```python
from build123d import *

# Parameters (mm, degrees)
BOSS_EXTRUDE1_DEPTH = 12
BOSS_EXTRUDE2_DEPTH = 13
SKETCH3_W           = 9
SKETCH3_H           = 12
BOSS_EXTRUDE3_DEPTH = 3.3
CUT_EXTRUDE1_DEPTH  = 34.256578297
CUT_EXTRUDE2_DEPTH  = 25.143114961
CUT_EXTRUDE3_DEPTH  = 25.143114961
CUT_EXTRUDE4_DEPTH  = 28.6007146
CUT_EXTRUDE5_DEPTH  = 28.748873851
CHAMFER1_SIZE       = 2.129646437


with BuildPart() as part:
    # Sketch1 → Boss-Extrude1 (new body)
    with BuildSketch(Plane.XZ.offset(17)):
        Polygon((16, 15), (3.3, 15), (3.3, 6), (11.968992121, -12.590713597), (16, -12.590713597), align=None)
    extrude(amount=-BOSS_EXTRUDE1_DEPTH)

    # Sketch2 → Boss-Extrude2 (add)
    with BuildSketch(Plane(origin=(0, -5, 0), x_dir=(-1, 0, 0), z_dir=(0, 1, 0))):
        Polygon((-16, 15), (-3.3, 15), (-3.3, 6), (-6.717465771, -1.328778996), (-13.611865759, -7.113867483), (-16, -4.267799921), align=None)
    extrude(amount=BOSS_EXTRUDE2_DEPTH)

    # Sketch3 → Boss-Extrude3 (add)
    with BuildSketch(Plane.ZY.offset(-3.3)):
        with Locations((10.5, -11)):
            Rectangle(SKETCH3_W, SKETCH3_H)
    extrude(amount=BOSS_EXTRUDE3_DEPTH)

    # Sketch4 → Cut-Extrude1 (cut, through all)
    with BuildSketch(Plane.XZ.offset(17)):
        Polygon((16, 15), (8.3, 15), (8.3, 3.870353563), (16, -2.590713597), align=None)
    extrude(amount=-CUT_EXTRUDE1_DEPTH, mode=Mode.SUBTRACT)

    # Sketch5 → Cut-Extrude2 (cut, through all)
    with BuildSketch(Plane(origin=(8.3, 0, 0), x_dir=(0, 0, -1), z_dir=(1, 0, 0))):
        with BuildLine():
            Line((-8.917452439, -10.971751585), (-10.5, -9.332975613))
            Line((-10.5, -9.332975613), (-12.082547561, -10.971751585))
            ThreePointArc((-12.082547561, -10.971751585), (-10.5, -14.7), (-8.917452439, -10.971751585))
        make_face()
    extrude(amount=-CUT_EXTRUDE2_DEPTH, mode=Mode.SUBTRACT)

    # Sketch6 → Cut-Extrude3 (cut, through all)
    with BuildSketch(Plane(origin=(8.3, 0, 0), x_dir=(0, 0, -1), z_dir=(1, 0, 0))):
        with BuildLine():
            Line((-8.917452439, 4.028248415), (-10.5, 5.667024387))
            Line((-10.5, 5.667024387), (-12.082547561, 4.028248415))
            ThreePointArc((-12.082547561, 4.028248415), (-10.5, 0.3), (-8.917452439, 4.028248415))
        make_face()
    extrude(amount=-CUT_EXTRUDE3_DEPTH, mode=Mode.SUBTRACT)

    # Sketch7 → Cut-Extrude4 (cut, through all)
    with BuildSketch(Plane(origin=(5.33513716, 0, 6.358168878), x_dir=(0.766044443118978, 0, -0.6427876096865394), z_dir=(0.6427876096865394, 0, 0.766044443118978))):
        with BuildLine():
            Line((12.082582782, 4.028248415), (10.500035221, 5.667024387))
            Line((10.500035221, 5.667024387), (8.91748766, 4.028248415))
            ThreePointArc((8.91748766, 4.028248415), (10.500035221, 0.3), (12.082582782, 4.028248415))
        make_face()
    extrude(amount=-CUT_EXTRUDE4_DEPTH, mode=Mode.SUBTRACT)

    # Sketch8 → Cut-Extrude5 (cut, through all)
    with BuildSketch(Plane(origin=(16, 0, 0), x_dir=(0, 0, -1), z_dir=(1, 0, 0))):
        with BuildLine():
            Line((9.852318341, -8.471751585), (8.26977078, -6.832975613))
            Line((8.26977078, -6.832975613), (6.68722322, -8.471751585))
            ThreePointArc((6.68722322, -8.471751585), (8.26977078, -12.2), (9.852318341, -8.471751585))
        make_face()
    extrude(amount=-CUT_EXTRUDE5_DEPTH, mode=Mode.SUBTRACT)

    # Chamfer1
    chamfer1_edges = [part.edges().sort_by_distance(p)[0] for p in [
        (8.3, -4.5, 3.870353563),
    ]]
    chamfer(chamfer1_edges, length=CHAMFER1_SIZE)


solid = part.part
```
Geometry check sheet. Reference: the model listing, model coordinates, mm. A direction names the side the tool comes from. Coordinates: 2 decimals unless noted, no trailing zeros. Write each loop counter-clockwise with the first axis right and the second up, starting at its lowest first coordinate (ties: lowest second). Pieces come first, ordered by that corner, then holes. Notation, with made-up numbers: M -26.5,37 L 4.5,37 A34 ccw 4.5,68 Z; hole C 84.5,15 d6. An arc over 180 degrees is marked long. Use one line per item in the form item = value. Start each with the question number.
1) Section check B-B on y = -3.75. Enter the section's corners in (x, z), and give its area (3 significant figures).
2) Thickness scan on probe 1 along Z at (x, y) = (12, -10); probe 2 along X at (y, z) = (-13.5, 8); probe 3 along Z at (x, y) = (11.5, -8.5). Record the ranges inside material, lowest first. Write a range as from..to.
3) Section check D-D on y = -13.75. Enter the section's corners in (x, z).
4) Go/stop test with flat-tipped pins: pin 1 Ø4.5 at (y, z) = (3.5, 9) entering from -X; pin 2 Ø1 at (x, y) = (5, 4.5) entering from -Z; pin 3 Ø3 at (x, z) = (12, -10) entering from +Y; pin 4 Ø3.5 at (y, z) = (-10, -8.27) entering from -X. Record where each tip stops, or that it passes through.
5) Release check for a two-part mould opening along Y. For faces 1 (the flat face through (4.21, -10.14, 11.28)), 2 (the flat face through (8, 8, 4)), 3 (the flat face through (0, -9.6, 11.4)) record: pulls with the +Y half, pulls with the -Y half, needs draft (parallel to the pull), parting line crosses it, or undercut.
6) Section check A-A on x = 3.75. Enter the section's corners in (y, z).
7) Section check C-C on y = 1. Enter the section's corners in (x, z).
8) Set-up check for faces 4 (the flat face through (14.8, 1.4, -5.7)), 5 (the flat face through (5.84, 4.84, 9.7)), 6 (the flat face through (2, -11, 6)): record each of +Z, -Z, +X, -X, +Y, -Y from which the full face is reachable in a straight line by a thin tool's end or side.
Responses:
q1.outline = M 3.3,6 L 6.72,-1.33 L 13.61,-7.11 L 16,-4.27 L 16,-2.59 L 9.93,2.5 L 8.3,6 L 8.3,15 L 3.3,15 Z
q1.area = 116 mm2
q2.probe_1 = -12.59..-10.47, -6.07..0.77
q2.probe_2 = 0..8.3
q2.probe_3 = -11.58..-9.88, -6.66..1.19
q3.outline = M 0,6 L 3.3,6 L 11.97,-12.59 L 16,-12.59 L 16,-2.59 L 9.93,2.5 L 8.3,6 L 8.3,8.69 L 0,8.69 Z; M 0,12.31 L 8.3,12.31 L 8.3,15 L 0,15 Z
q4.pin_1 = 3.3
q4.pin_2 = 1.28
q4.pin_3 = -5
q4.pin_4 = through
q5.face_1 = undercut
q5.face_2 = pulls with the +Y half
q5.face_3 = needs draft
q6.outline = M -17,5.03 L 8,5.03 L 8,15 L -17,15 Z; hole M -10.97,8.92 L -9.33,10.5 L -10.97,12.08 A2.2 ccw long Z; hole M 4.03,8.92 L 5.67,10.5 L 4.03,12.08 A2.2 ccw long Z
q7.outline = M 3.3,6 L 6.72,-1.33 L 8.93,-3.19 L 12.15,0.64 L 9.93,2.5 L 8.3,6 L 8.3,8.89 L 3.3,8.89 Z; M 3.3,12.11 L 8.3,12.11 L 8.3,15 L 3.3,15 Z; M 11.4,-5.26 L 13.61,-7.11 L 16,-4.27 L 16,-2.59 L 14.61,-1.43 Z
q8.face_4 = -Z, +X, +Y
q8.face_5 = +X, -X
q8.face_6 = -Z, -X, +Y, -Y
